Check sheet for the modelled part. Datum: model origin and axes. Units: mm. Round coordinates to 2 decimals unless told otherwise and drop trailing zeros. Loops run counter-clockwise (first coordinate to the right, second up) from the corner with the lowest first, then second, coordinate; pieces in that order, holes last. Notation, with made-up numbers: (-7.75, -0.5) -> (13.25, -0.5) arc R27 ccw to (13.25, 23.5) -> close; hole circle Ø3 at (37.5, 76). An arc over 180 degrees is marked (long way). Use one line per item in the form item = value. Start each with the question number.
(1) Go/stop test with flat-tipped pins: pin 1 (1.5 mm diameter, centred on x = 204.5, z = 1, fed in from -Y); pin 2 (1.5 mm diameter, centred on y = -2, z = 1, fed in from -X). Record where each tip stops, or that it passes through.
(2) Material ranges on probe 1 along X at (y, z) = (18.5, 0.1); probe 2 along X at (y, z) = (-1, 1.9); probe 3 along Y at (x, z) = (27, 2.1), recorded low to high. Write a range as [from, to].
(3) Sectioned sample at A-A (z = 1.7). Record the cut outline in (x, y), and give its area (4 significant figures).
(4) Sectioned sample at C-C (x = 30). Record the cut outline in (y, z), and give its area (3 significant figures).
(5) Sectioned sample at B-B (y = 15). Record the cut outline in (x, z), and give its area (4 significant figures).
from build123d import *

# Parameters (mm, degrees)
SKETCH_1_W      = 20
SKETCH_1_H      = 3
EXTRUDE_1_DEPTH = 3


with BuildPart() as part:
    # 草图1 → 凸台-拉伸1 (new body)
    with BuildSketch(Plane.XY):
        Polygon((-2.75, 0), (0, 0), (20, 0), (180, 0), (200, 0), (202.75, 0), (207.75, 0), (207.75, 30), (202.75, 30), (200, 30), (0, 30), (-2.75, 30), (-7.75, 30), (-7.75, 0), align=None)
        Polygon((-2.75, 22.5), (-2.75, 15), (-2.75, 7.5), (-5.75, 7.5), (-5.75, 22.5), align=None, mode=Mode.SUBTRACT)
        Polygon((202.75, 7.5), (202.75, 15), (202.75, 22.5), (205.75, 22.5), (205.75, 7.5), align=None, mode=Mode.SUBTRACT)
        with Locations((10, -1.5)):
            Rectangle(SKETCH_1_W, SKETCH_1_H)
        with Locations((190, -1.5)):
            Rectangle(SKETCH_1_W, SKETCH_1_H)
    extrude(amount=EXTRUDE_1_DEPTH)


solid = part.part
Checks:
q1.pin_1 = 0
q1.pin_2 = 0
q2.probe_1 = [-7.75, -5.75], [-2.75, 202.75], [205.75, 207.75]
q2.probe_2 = [0, 20], [180, 200]
q2.probe_3 = [0, 30]
q3.outline = (-7.75, 0) -> (0, 0) -> (0, -3) -> (20, -3) -> (20, 0) -> (180, 0) -> (180, -3) -> (200, -3) -> (200, 0) -> (207.75, 0) -> (207.75, 30) -> (-7.75, 30) -> close; hole (-5.75, 7.5) -> (-2.75, 7.5) -> (-2.75, 22.5) -> (-5.75, 22.5) -> close; hole (202.75, 7.5) -> (205.75, 7.5) -> (205.75, 22.5) -> (202.75, 22.5) -> close
q3.area = 6,495 mm2
q4.outline = (0, 0) -> (30, 0) -> (30, 3) -> (0, 3) -> close
q4.area = 90.0 mm2
q5.outline = (-7.75, 0) -> (-5.75, 0) -> (-5.75, 3) -> (-7.75, 3) -> close; (-2.75, 0) -> (202.75, 0) -> (202.75, 3) -> (-2.75, 3) -> close; (205.75, 0) -> (207.75, 0) -> (207.75, 3) -> (205.75, 3) -> close
q5.area = 628.5 mm2
